Geometry: final body of the model. Coordinates: model frame, mm. A direction names the side the tool comes from. Give positions to 0.01 mm unless a question says otherwise; leave off trailing zeros. Write each loop counter-clockwise with the first axis right and the second up, starting at its lowest first coordinate (ties: lowest second). Pieces come first, ordered by that corner, then holes.
```python
from build123d import *

# Parameters (mm, degrees)
SKETCH1_R           = 9
SKETCH1_R_2         = 5.5
BOSS_EXTRUDE1_DEPTH = 3
SKETCH2_R           = 13
SKETCH2_R_2         = 5.5
BOSS_EXTRUDE2_DEPTH = 3
SKETCH3_R           = 1
SKETCH3_R_2         = 2.5
CUT_EXTRUDE1_DEPTH  = 20.339079606
CHAMFER1_SIZE       = 2


with BuildPart() as part:
    # Sketch1 → Boss-Extrude1 (new body)
    with BuildSketch(Plane(origin=(0, 0, 0), x_dir=(0, 0, -1), z_dir=(1, 0, 0))):
        Circle(SKETCH1_R)
        Circle(SKETCH1_R_2, mode=Mode.SUBTRACT)
    extrude(amount=BOSS_EXTRUDE1_DEPTH)

    # Sketch2 → Boss-Extrude2 (add)
    with BuildSketch(Plane(origin=(3, 0, 0), x_dir=(0, 0, -1), z_dir=(1, 0, 0))):
        Circle(SKETCH2_R)
        Circle(SKETCH2_R_2, mode=Mode.SUBTRACT)
    extrude(amount=BOSS_EXTRUDE2_DEPTH)

    # Sketch3 → Cut-Extrude1 (cut, through all)
    with BuildSketch(Plane(origin=(6, 0, 0), x_dir=(0, 0, -1), z_dir=(1, 0, 0))):
        with Locations((7.919595949, 7.919595949)):
            Circle(SKETCH3_R)
        with Locations((7.919595949, -7.919595949)):
            Circle(SKETCH3_R)
        with Locations((-7.919595949, -7.919595949)):
            Circle(SKETCH3_R)
        with Locations((-7.919595949, 7.919595949)):
            Circle(SKETCH3_R)
        with Locations((0, 13)):
            Circle(SKETCH3_R_2)
        with Locations((13, 0)):
            Circle(SKETCH3_R_2)
        with Locations((0, -13)):
            Circle(SKETCH3_R_2)
        with Locations((-13, 0)):
            Circle(SKETCH3_R_2)
    extrude(amount=-CUT_EXTRUDE1_DEPTH, mode=Mode.SUBTRACT)

    # Chamfer1
    chamfer1_edges = [part.edges().sort_by_distance(p)[0] for p in [
        (6, 0, 5.5),
    ]]
    chamfer(chamfer1_edges, length=CHAMFER1_SIZE)


solid = part.part
```
Item 1: Line query: L1, parallel to Y at x = 2, z = 0; L2, parallel to Z at x = 1.65, y = -5; L3, parallel to Y at x = 1.2, z = -1.75. Output: solid intervals per line, ascending.
Found:
L1: y = -9 to -5.5, 5.5 to 9
L2: z = -7.48 to -2.29, 2.29 to 7.48
L3: y = -8.83 to -5.21, 5.21 to 8.83
Item 2: Reachability of faces 1 (the face through (1.479, 8.923, 1.172)), 2 (the face through (4.479, -9.268, -9.116)) from +Z, -Z, +X, -X, +Y, -Y: full face, straight path, thin tool, end or side. Return the list, or none.
Found:
face 1: -X
face 2: -Z, +X, -X, -Y
Item 3: Pull-direction query (Y, two-part tool) for faces 3 (the face through (3, -3, 9)), 4 (the face through (1.97, -5.37, 1.19)), 5 (the face through (4.479, -9.116, 9.268)), 6 (the face through (4.521, 8.22, -8.873)); classes: +Y half, -Y half, draft (parallel to the pull), parting line (faces both ways), or undercut.
Found:
face 3: draft
face 4: undercut
face 5: -Y half
face 6: undercut
Item 4: Section A-A, the plane z = 0. Return the cut outline in (x, y).
Found:
outline: (0, -9) - (3, -9) - (3, -10.5) - (6, -10.5) - (6, -7.5) - (4, -5.5) - (0, -5.5) - close; (0, 5.5) - (4, 5.5) - (6, 7.5) - (6, 10.5) - (3, 10.5) - (3, 9) - (0, 9) - close
Item 5: Pin query (flat end, axial travel): pin 1 Ø1.5 at (x, y) = (4, 7.5) entering from +Z; pin 2 Ø1.2 at (y, z) = (-7.92, -7.92) entering from +X; pin 3 Ø2.5 at (y, z) = (7.92, -7.92) entering from -X; pin 4 Ø2 at (x, y) = (3.5, -6) entering from -Z. Return the tip coordinate at first contact, or that it passes through.
Found:
pin 1: stops at z = 11.11
pin 2: passes through
pin 3: stops at x = 3
pin 4: stops at z = -12
Item 6: Section D-D, the plane x = 4.85. Return the cut outline in (y, z).
Found:
outline: (-12.76, -2.49) arc R13 ccw to (-2.49, -12.76) arc R2.5 cw to (2.49, -12.76) arc R13 ccw to (12.76, -2.49) arc R2.5 cw to (12.76, 2.49) arc R13 ccw to (2.49, 12.76) arc R2.5 cw to (-2.49, 12.76) arc R13 ccw to (-12.76, 2.49) arc R2.5 cw to start; hole circle Ø2 at (-7.92, -7.92); hole circle Ø2 at (-7.92, 7.92); hole circle Ø12.7 at (0, 0); hole circle Ø2 at (7.92, -7.92); hole circle Ø2 at (7.92, 7.92)
Item 7: Section C-C, the plane x = 0.5. Return the cut outline in (y, z).
Found:
outline: circle Ø18 at (0, 0); hole circle Ø11 at (0, 0)
